```python
from build123d import *

# Parameters (mm, degrees)
CROQUIS1_R              = 1.5
CROQUIS1_W              = 30
CROQUIS1_H              = 30
SALIENTE_EXTRUIR1_DEPTH = 1


with BuildPart() as part:
    # Croquis1 → Saliente-Extruir1 (new body)
    with BuildSketch(Plane(origin=(0, 0, 0), x_dir=(1, 0, 0), z_dir=(0, 1, 0))):
        with BuildLine():
            Line((-5, 30.550343704), (-5, -0.550343704))
            ThreePointArc((-5, -0.550343704), (-5.850097081, -2.836828892), (-7.987436867, -4.012608719))
            ThreePointArc((-7.987436867, -4.012608719), (-9.949747468, -9.949747468), (-4.012608719, -7.987436867))
            ThreePointArc((-4.012608719, -7.987436867), (-2.836828892, -5.850097081), (-0.550343704, -5))
            Line((-0.550343704, -5), (30.550343704, -5))
            ThreePointArc((30.550343704, -5), (32.836828892, -5.850097081), (34.012608719, -7.987436867))
            ThreePointArc((34.012608719, -7.987436867), (39.949747468, -9.949747468), (37.987436867, -4.012608719))
            ThreePointArc((37.987436867, -4.012608719), (35.850097081, -2.836828892), (35, -0.550343704))
            Line((35, -0.550343704), (35, 30.550343704))
            ThreePointArc((35, 30.550343704), (35.850097081, 32.836828892), (37.987436867, 34.012608719))
            ThreePointArc((37.987436867, 34.012608719), (39.949747468, 39.949747468), (34.012608719, 37.987436867))
            ThreePointArc((34.012608719, 37.987436867), (32.836828892, 35.850097081), (30.550343704, 35))
            Line((30.550343704, 35), (-0.550343704, 35))
            ThreePointArc((-0.550343704, 35), (-2.836828892, 35.850097081), (-4.012608719, 37.987436867))
            ThreePointArc((-4.012608719, 37.987436867), (-9.949747468, 39.949747468), (-7.987436867, 34.012608719))
            ThreePointArc((-7.987436867, 34.012608719), (-5.850097081, 32.836828892), (-5, 30.550343704))
        make_face()
        with Locations(Location((7, -2.5, 0), (0, 0, 270))):
            Circle(CROQUIS1_R, mode=Mode.SUBTRACT)
        with Locations(Location((15, -2.5, 0), (0, 0, 270))):
            Circle(CROQUIS1_R, mode=Mode.SUBTRACT)
        with Locations(Location((-2.5, 7, 0), (0, 0, 270))):
            Circle(CROQUIS1_R, mode=Mode.SUBTRACT)
        with Locations((15, 15)):
            Rectangle(CROQUIS1_W, CROQUIS1_H, mode=Mode.SUBTRACT)
        with Locations(Location((23, -2.5, 0), (0, 0, 270))):
            Circle(CROQUIS1_R, mode=Mode.SUBTRACT)
        with Locations(Location((32.5, 7, 0), (0, 0, 270))):
            Circle(CROQUIS1_R, mode=Mode.SUBTRACT)
        with Locations(Location((32.5, 15, 0), (0, 0, 270))):
            Circle(CROQUIS1_R, mode=Mode.SUBTRACT)
        with Locations(Location((-2.5, 15, 0), (0, 0, 270))):
            Circle(CROQUIS1_R, mode=Mode.SUBTRACT)
        with Locations(Location((-2.5, 23, 0), (0, 0, 270))):
            Circle(CROQUIS1_R, mode=Mode.SUBTRACT)
        with Locations(Location((-7.474873734, 37.474873734, 0), (0, 0, 270))):
            Circle(CROQUIS1_R, mode=Mode.SUBTRACT)
        with Locations(Location((7, 32.5, 0), (0, 0, 270))):
            Circle(CROQUIS1_R, mode=Mode.SUBTRACT)
        with Locations(Location((32.5, 23, 0), (0, 0, 270))):
            Circle(CROQUIS1_R, mode=Mode.SUBTRACT)
        with Locations(Location((15, 32.5, 0), (0, 0, 270))):
            Circle(CROQUIS1_R, mode=Mode.SUBTRACT)
        with Locations(Location((23, 32.5, 0), (0, 0, 270))):
            Circle(CROQUIS1_R, mode=Mode.SUBTRACT)
        with Locations(Location((-7.474873734, -7.474873734, 0), (0, 0, 270))):
            Circle(CROQUIS1_R, mode=Mode.SUBTRACT)
        with Locations(Location((37.474873734, -7.474873734, 0), (0, 0, 270))):
            Circle(CROQUIS1_R, mode=Mode.SUBTRACT)
        with Locations(Location((37.474873734, 37.474873734, 0), (0, 0, 270))):
            Circle(CROQUIS1_R, mode=Mode.SUBTRACT)
    extrude(amount=SALIENTE_EXTRUIR1_DEPTH)


solid = part.part
```
Could you check a few things on this model? Use its own coordinates, in mm. Coordinates: 2 decimals unless noted, no trailing zeros. Loops run counter-clockwise (first coordinate to the right, second up) from the corner with the lowest first, then second, coordinate; pieces in that order, holes last.
1) Thinking about a two-plate mould opening in X: for faces 1 (the face through (17, 1, -31)), 2 (the face through (-2.43, 0.49, -24.5)), which applies, released by +X, released by -X, zero draft, split by the parting line, or undercut?
Reported:
face 1: zero draft
face 2: undercut
2) Will this pin go through, and if not, where does the flat tip stop? pin 1 Ø4 at (x, z) = (-7.47, -37.47) entering from -Y.
Reported:
pin 1: stops at y = 0
3) Imagine slicing it at D-D (x = 32.5). List the corners of the cut face in (y, z) for me.
Reported:
outline: (0, -35.59) - (1, -35.59) - (1, -24.5) - (0, -24.5) - close; (0, -21.5) - (1, -21.5) - (1, -16.5) - (0, -16.5) - close; (0, -13.5) - (1, -13.5) - (1, -8.5) - (0, -8.5) - close; (0, -5.5) - (1, -5.5) - (1, 5.59) - (0, 5.59) - close
4) Please list where these lines run through material, in increasing order: line 1 along X through (y, z) = (0.4, -7); line 2 along X through (y, z) = (0.9, -22.5); line 3 along X through (y, z) = (0.5, -17).
Reported:
line 1: x = -5 to -4, -1 to 0, 30 to 31, 34 to 35
line 2: x = -5 to -3.91, -1.09 to 0, 30 to 31.09, 33.91 to 35
line 3: x = -5 to 0, 30 to 35
5) Imagine slicing it at C-C (y = 0.25). State how many separate pieces and enclosed holes the cut face has, and give its area (3 significant figures).
Reported:
separate pieces: 1
enclosed holes: 17
area: 766 mm2
6) Imagine slicing it at A-A (z = -10.5). List the corners of the cut face in (x, y) for me, and give its area (3 significant figures).
Reported:
outline: (-5, 0) - (0, 0) - (0, 1) - (-5, 1) - close; (30, 0) - (35, 0) - (35, 1) - (30, 1) - close
area: 10.0 mm2
7) Imagine slicing it at B-B (x = 7). List the corners of the cut face in (y, z) for me, and give its area (3 significant figures).
Reported:
outline: (0, -35) - (1, -35) - (1, -34) - (0, -34) - close; (0, -31) - (1, -31) - (1, -30) - (0, -30) - close; (0, 0) - (1, 0) - (1, 1) - (0, 1) - close; (0, 4) - (1, 4) - (1, 5) - (0, 5) - close
area: 4.00 mm2
